from build123d import *

# Parameters (mm, degrees)
F1_DEPTH  = 10
F2_R      = 7.5
F3_DEPTH  = 4.8
F4_R      = 1.9
F5_DEPTH  = 25
F6_R      = 1.9
F7_DEPTH  = 7
F9_R      = 7.5
F10_DEPTH = 4.5
F11_R     = 1.9
F12_DEPTH = 25
F13_R     = 1.9
F14_DEPTH = 25


with BuildPart() as f1:
    # F0 (on Front) → F1 (new body)
    with BuildSketch(Plane.XZ):
        with BuildLine():
            Line((-37.2161355778, 126.6291381083), (-51.2161355778, 126.6291381083))
            ThreePointArc((-51.2161355778, 126.6291381083), (-55.4587762649, 124.8717787955), (-57.2161355778, 120.6291381083))
            Line((-57.2161355778, 120.6291381083), (-57.2161355778, 12.6291381083))
            ThreePointArc((-57.2161355778, 12.6291381083), (-55.4587762649, 8.3864974212), (-51.2161355778, 6.6291381083))
            Line((-51.2161355778, 6.6291381083), (-43.2161355778, 6.6291381083))
            ThreePointArc((-43.2161355778, 6.6291381083), (-38.9734948907, 8.3864974212), (-37.2161355778, 12.6291381083))
            Line((-37.2161355778, 12.6291381083), (-37.2161355778, 126.6291381083))
        make_face()
    extrude(amount=F1_DEPTH)

    # F2 (on face) → F3 (join)
    with BuildSketch(Plane.XY.offset(126.6291381083)):
        with Locations((-31.6986439976, -4.9055621816)):
            Circle(F2_R)
    extrude(amount=-F3_DEPTH)

    # F4 (on face) → F5 (cut)
    with BuildSketch(Plane.XY.offset(126.6291381083)):
        with Locations((-31.6986439976, -4.9055621816)):
            Circle(F4_R)
    extrude(amount=-F5_DEPTH, mode=Mode.SUBTRACT)

    # F6 (on face) → F7 (cut)
    with BuildSketch(Plane(origin=(-57.2161355778, 0, 0), x_dir=(0, -1, 0), z_dir=(-1, 0, 0))):
        with Locations((5, 38.5266803205)):
            Circle(F6_R)
        with Locations((5, 12.2715812176)):
            Circle(F6_R)
    extrude(amount=-F7_DEPTH, mode=Mode.SUBTRACT)

    # F9 (on offset) → F10 (join)
    with BuildSketch(Plane.XY.offset(86.6291381083)):
        with Locations((-31.6911898553, -5.0173136406)):
            Circle(F9_R)
    extrude(amount=F10_DEPTH)

    # F11 (on face) → F12 (cut)
    with BuildSketch(Plane.XY.offset(91.1291381083)):
        with Locations((-31.6911898553, -5.0173136406)):
            Circle(F11_R)
    extrude(amount=-F12_DEPTH, mode=Mode.SUBTRACT)

    # F13 (on face) → F14 (cut)
    with BuildSketch(Plane(origin=(0, 0, 0), x_dir=(-1, 0, 0), z_dir=(0, 1, 0))):
        with Locations((47.2161355778, 81.6291381083)):
            Circle(F13_R)
        with Locations((47.2161355778, 74.6291381083)):
            Circle(F13_R)
        with Locations((47.2161355778, 53.6291381083)):
            Circle(F13_R)
        with Locations((47.2161355778, 67.6291381083)):
            Circle(F13_R)
        with Locations((47.2161355778, 60.6291381083)):
            Circle(F13_R)
        with Locations((47.2161355778, 18.6291381083)):
            Circle(F13_R)
        with Locations((47.2161355778, 25.6291381083)):
            Circle(F13_R)
        with Locations((47.2161355778, 32.6291381083)):
            Circle(F13_R)
        with Locations((47.2161355778, 39.6291381083)):
            Circle(F13_R)
        with Locations((47.2161355778, 46.6291381083)):
            Circle(F13_R)
        with Locations((47.2161355778, 11.6291381083)):
            Circle(F13_R)
    extrude(amount=-F14_DEPTH, mode=Mode.SUBTRACT)


solid = f1.part
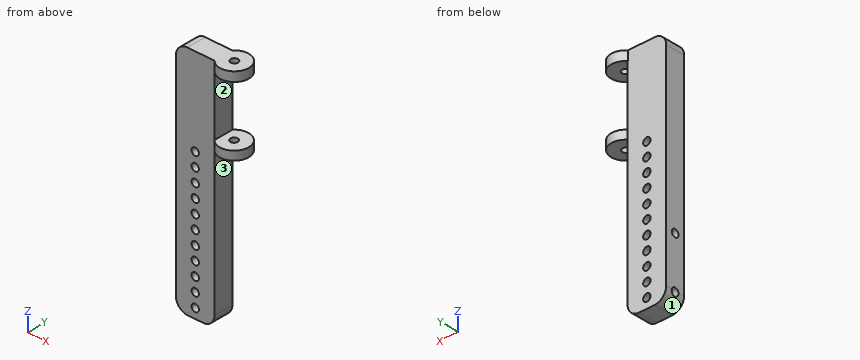
Source: CAD feature listing. Evaluate the final solid. Frame: model axes, mm. Face numbers are marked on the shaded views. Coordinates: 2 decimals unless noted, no trailing zeros. Loops run counter-clockwise (first coordinate to the right, second up) from the corner with the lowest first, then second, coordinate; pieces in that order, holes last. Notation, with made-up numbers: (-33, 83.25) - (23, 83.25) arc R14 ccw to (23, 98.25) - close; hole circle Ø5 at (-11.75, 56). An arc over 180 degrees is marked (long way). Return JSON: item names as keys, results as strings.
Q1. Section B-B, the plane z = 106. Return loops of the section in (x, y).
Results:
{"outline": "(-57.22, -10) - (-37.22, -10) - (-37.22, 0) - (-57.22, 0) - close"}
Q2. Mould query, pull axis Z, two halves, no side actions, for the marked faces 1, 2 and 3. Classes: released by +Z, released by -Z, zero draft, split by the parting line, or undercut.
Results:
{"face 1": "released by -Z", "face 2": "undercut", "face 3": "zero draft"}
Q3. Contact query for flat-ended pins moving along their axis: P1, Ø10, axis at x = -52, z = 53.5, coming from the -Y side; P2, Ø4.5, axis at x = -31.7, y = -4.91, coming from the +Z side; P3, Ø1, axis at x = -27.5, z = 89, coming from the +Y side; P4, Ø6, axis at x = -47.22, z = 32.63, coming from the +Y side. Output: stop coordinate, or through.
Results:
{"P1": "y = -10", "P2": "z = 126.63", "P3": "y = 1.51", "P4": "y = 0"}
Q4. Material intervals for line 1 along Z through (x, y) = (-55, -5); line 2 along Y through (x, z) = (-43.5, 26.5); line 3 along Z through (x, y) = (-30, -8), sorted ascending.
Results:
{"line 1": "7.97 to 10.37, 14.17 to 36.63, 40.43 to 125.29", "line 2": "-10 to 0", "line 3": "86.63 to 91.13, 121.83 to 126.63"}
Q5. Section A-A, the plane y = -2. Give the number of separate pieces and of enclosed holes in the cut face, plus the area to 3 significant figures.
Results:
{"separate pieces": "1", "enclosed holes": "11", "area": "2,370 mm2"}
